Autodesk Inventor part; units mm, degrees
ref_plane "YZ Plane" through (0, 0, 0) normal (1, 0, 0) x (0, 1, 0)
ref_plane "XZ Plane" through (0, 0, 0) normal (0, 1, 0) x (-1, 0, 0)
ref_plane "XY Plane" through (0, 0, 0) normal (0, 0, 1) x (1, 0, 0)
sketch "Sketch1" plane through (0, 0, 0) normal (0, 1, 0) x (-1, 0, 0)
  line L0 (0, 0) -> (17.3, 0)
  line L1 (17.3, 0) -> (17.3, -2.8)
  line L2 (0, 0) -> (0, -19.8)
  line L3 (7.3, -17.3) -> (2.8, -17.3)
  line L4 (2.8, -17.3) -> (2.8, -2.8)
  line L5 (2.8, -2.8) -> (17.3, -2.8)
  arc A0 (17.3, -17.3) -> (7.3, -17.3) centre (12.3, -23.3444) ccw
  line L6 (7.3, -17.3) -> (18.5004, -17.3) construction
  line L7 (17.3, -17.3) -> (17.3, -19.3)
  line L8 (17.3, -19.3) -> (0, -19.8)
  point P0 (12.3, -15.5)
  dimension "d1" = 2.8
  dimension "d3" = 2.8
  dimension "d11" = 10
  dimension "d12" = 4.5
  dimension "d13" = 14.5
  dimension "d19" = 2
  dimension "d20" = 19.8
  dimension "d22" = 1.8
extrude "Extrusion1" add sketch "Sketch1" along normal blind 2.6
properties part number "Cuvette_retainer"
For this review, take the finished solid that the model builds, in its own axes (mm). A direction names the side the tool comes from. Round coordinates to 2 decimals unless told otherwise and drop trailing zeros. Loops run counter-clockwise (first coordinate to the right, second up) from the corner with the lowest first, then second, coordinate; pieces in that order, holes last. Notation, with made-up numbers: (-15.5, -40) - (17.5, -40) arc R23 ccw to (17.5, -18) - close; hole circle Ø2 at (-19.75, -39). An arc over 180 degrees is marked (long way). One line per item, written item: value. Start each with the question number.
Item 1: Clearance check with flat-ended pins moving along their axes: pin 1 Ø5 at (x, z) = (-5, -9.5) entering from +Y; pin 2 Ø3 at (x, z) = (-5.5, -7) entering from +Y; pin 3 Ø1 at (y, z) = (0.5, -7.5) entering from -X. State where each tip first meets the part, or that it passes through.
Item 2: Take a section at D-D (z = -7). Give the boundary of the cut face in (x, y), plus the area to 3 significant figures.
Item 3: Take a section at A-A (x = -15.5). Give the boundary of the cut face in (y, z), plus the area to 3 significant figures.
Item 4: The part is to be moulded in two halves that separate along X. For faces 1 (the flat face through (-9, 1, 0)), 2 (the cylindrical face through (-12.2, 1.3, -15.5)), 3 (the flat face through (-17.3, 1, -18)), 4 (the flat face through (-5, 1, -17.3)), say which applies: +X half, -X half, draft (parallel to the pull), parting line (faces both ways), or undercut.
Item 5: Take a section at B-B (y = 0.9). Give the boundary of the cut face in (x, z), plus the area to 3 significant figures.
Item 6: For faces 5 (the flat face through (-1, 0, -10)), 6 (the flat face through (-10, 1, -2.8)), list the 3-axis set-ups (+Z, -Z, +X, -X, +Y, -Y) from which the entire face can be reached by the end or side of a thin tool; tool diameter is ignored.
Item 7: For L1, parallel to X at y = 0.45, z = -13.5; L2, parallel to Z at x = -12.5, y = 2.05; L3, parallel to Z at x = -10, y = 2.55, list the stretches that pass through material, from the lowest coordinate up.
Item 8: Take a section at C-C (z = -16.5). Give the boundary of the cut face in (x, y).
Answer below:
1. pin 1: stops at y = 2.6
1. pin 2: passes through
1. pin 3: stops at x = -2.8
2. outline: (-2.8, 0) - (0, 0) - (0, 2.6) - (-2.8, 2.6) - close
2. area: 7.28 mm2
3. outline: (0, -19.35) - (2.6, -19.35) - (2.6, -16.18) - (0, -16.18) - close; (0, -2.8) - (2.6, -2.8) - (2.6, 0) - (0, 0) - close
3. area: 15.5 mm2
4. face 1: draft
4. face 2: undercut
4. face 3: -X half
4. face 4: undercut
5. outline: (-17.3, -19.3) - (0, -19.8) - (0, 0) - (-17.3, 0) - (-17.3, -2.8) - (-2.8, -2.8) - (-2.8, -17.3) - (-7.3, -17.3) arc R7.84 ccw to (-17.3, -17.3) - close
5. area: 140 mm2
6. face 5: +Z, -Z, +X, -X, -Y
6. face 6: -X, +Y, -Y
7. L1: x = -2.8 to 0
7. L2: z = -19.44 to -15.5, -2.8 to 0
7. L3: z = -19.51 to -15.84, -2.8 to 0
8. outline: (-16.13, 0) - (-8.47, 0) - (-8.47, 2.6) - (-16.13, 2.6) - close; (-2.8, 0) - (0, 0) - (0, 2.6) - (-2.8, 2.6) - close
